```python
from build123d import *

# Parameters (mm, degrees)
F2_T = -0.9


with BuildPart() as f1:
    # F0 (on Front) → F1 (revolve)
    with BuildSketch(Plane.XZ):
        with BuildLine():
            Line((-6, 0), (0, 0))
            Line((0, 0), (0, 30))
            Line((0, 30), (-2.7065660749, 30))
            Line((-2.7065660749, 30), (-2.7065660749, 6.3329207692))
            Line((-2.7065660749, 6.3329207692), (-3.3541182942, 4.5065977652))
            ThreePointArc((-3.3541182942, 4.5065977652), (-3.804509639, 3.6790523714), (-4.4893614126, 3.0320115764))
            Line((-4.4893614126, 3.0320115764), (-6, 2))
            Line((-6, 2), (-6, 0))
        make_face()
    revolve(axis=Axis((0, 0, 15), (0, 0, 1)))

    # F2
    f2_openings = [f1.faces().sort_by_distance(p)[0] for p in [
        (0, 0, 30),
    ]]
    offset(amount=F2_T, openings=f2_openings, kind=Kind.INTERSECTION)


solid = f1.part
```
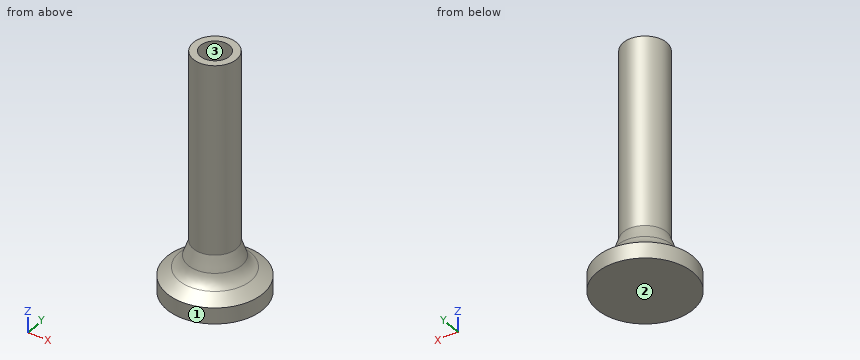
Geometry: final body of the model. Coordinates: model frame, mm. Face numbers are marked on the shaded views. Give positions to 0.01 mm unless a question says otherwise; leave off trailing zeros. Loops run counter-clockwise (first coordinate to the right, second up) from the corner with the lowest first, then second, coordinate; pieces in that order, holes last. Notation, with made-up numbers: (60, -11) - (90, -11) arc R15 ccw to (90, -4) - close; hole circle Ø4 at (11, 28.25). An arc over 180 degrees is marked (long way). Answer as CSV lines item,"result". Start each with the question number.
(1) Section query D-D (z = 2.75). Output: boundary loops of the cut face in (x, y), and give its area (3 significant figures).
(2) Mould query, pull axis X, two halves, no side actions, for the marked faces 1, 2 and 3. Classes: +X half, -X half, draft (parallel to the pull), parting line (faces both ways), or undercut.
(3) Section query A-A (x = 0). Output: boundary loops of the cut face in (y, z), and give its area (3 significant figures).
(4) Ray query, line 1 along Y through (x, z) = (0, 1.4); line 2 along X through (y, z) = (0, 17.25). Return the intervals inside material, ascending. Write a range as [from, to].
(5) Pin query (flat end, axial travel): P1, Ø5, axis at x = -1.5, y = -2, coming from the -Z side; P2, Ø1, axis at x = -2, z = 3.5, coming from the +Y side; P3, Ø6, axis at y = 2, z = 13.5, coming from the +X side; P4, Ø3, axis at x = 0, y = 0, coming from the +Z side. Return the tip coordinate at first contact, or that it passes through.
(6) Section query C-C (z = 23.25). Output: boundary loops of the cut face in (x, y), and give its area (3 significant figures).
Worked answers:
1,outline,"circle Ø9.8 at (0, 0); hole circle Ø6.85 at (0, 0)"
1,area,"38.6 mm^2"
2,face 1,"parting line"
2,face 2,"draft"
2,face 3,"undercut"
3,outline,"(-6, 0) - (6, 0) - (6, 2) - (4.49, 3.03) arc R3 cw to (3.35, 4.51) - (2.71, 6.33) - (2.71, 30) - (1.81, 30) - (1.81, 6.18) - (2.51, 4.21) arc R3.9 ccw to (3.98, 2.29) - (5.1, 1.52) - (5.1, 0.9) - (-5.1, 0.9) - (-5.1, 1.52) - (-3.98, 2.29) arc R3.9 ccw to (-2.51, 4.21) - (-1.81, 6.18) - (-1.81, 30) - (-2.71, 30) - (-2.71, 6.33) - (-3.35, 4.51) arc R3 cw to (-4.49, 3.03) - (-6, 2) - close"
3,area,"65.5 mm^2"
4,line 1,"y = [-6, -5.1], [5.1, 6]"
4,line 2,"x = [-2.71, -1.81], [1.81, 2.71]"
5,P1,"stops at z = 0"
5,P2,"stops at y = 4.11"
5,P3,"stops at x = 2.71"
5,P4,"stops at z = 0.9"
6,outline,"circle Ø5.41 at (0, 0); hole circle Ø3.61 at (0, 0)"
6,area,"12.8 mm^2"
